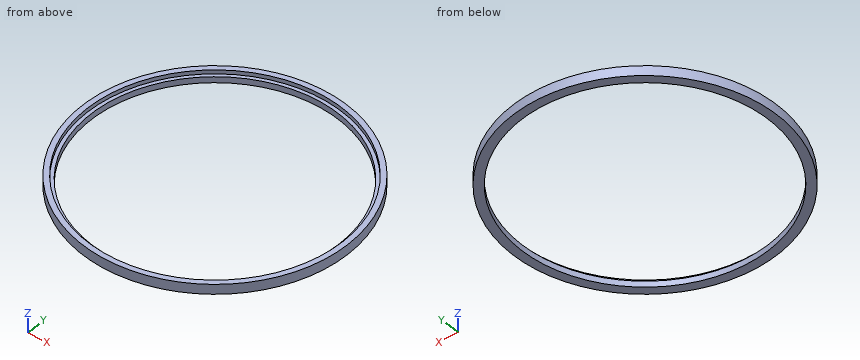
```python
from build123d import *

# Parameters (mm, degrees)
F0_R     = 67
F0_R_2   = 64.375
F1_DEPTH = 5
F0_R_3   = 62.625
F2_DEPTH = 3
F0_R_4   = 58.875
F3_DEPTH = 2
F4_R     = 5.75
F5_DEPTH = 192


# Not quite as in the source:
# - an extrude ends at something that could not be found from the text; its depth is read off the source's solid


with BuildPart() as f1:
    # F0 (on Top) → F1 (new body)
    with BuildSketch(Plane.XY):
        Circle(F0_R)
        Circle(F0_R_2, mode=Mode.SUBTRACT)
    extrude(amount=F1_DEPTH)

    # F0 (on Top) → F2 (join)
    with BuildSketch(Plane.XY):
        Circle(F0_R_2)
        Circle(F0_R_3, mode=Mode.SUBTRACT)
    extrude(amount=F2_DEPTH)

    # F0 (on Top) → F3 (cut)
    with BuildSketch(Plane.XY):
        Circle(F0_R_3)
        Circle(F0_R_4, mode=Mode.SUBTRACT)
    extrude(amount=F3_DEPTH, mode=Mode.SUBTRACT)

    # F4 (on Top) → F5 (cut, through all)
    with BuildSketch(Plane.XY):
        with Locations((0, 46.25)):
            Circle(F4_R)
    extrude(amount=-F5_DEPTH, mode=Mode.SUBTRACT)


solid = f1.part
```
Can you work these out from the model? Positions are in its coordinate system, mm. Coordinates: 2 decimals unless noted, no trailing zeros. Loops run counter-clockwise (first coordinate to the right, second up) from the corner with the lowest first, then second, coordinate; pieces in that order, holes last. Notation, with made-up numbers: (-26.5, 3) -> (14.5, 3) arc R16 ccw to (14.5, 11) -> close; hole circle Ø4 at (28.25, 39.5). An arc over 180 degrees is marked (long way). Answer as a JSON object with one key per item and string values.
1) Imagine slicing it at C-C (z = 1.55). Please give me the cut outline in (x, y) (3 decimals), then the cut area to 3 significant figures.
Results:
{"outline": "circle Ø134 at (0, 0); hole circle Ø125.25 at (0, 0)", "area": "1,780 mm^2"}
2) Imagine slicing it at A-A (x = 0). Please give me the cut outline in (y, z) (3 decimals), then the cut area to 4 significant figures.
Results:
{"outline": "(-67, 0) -> (-62.625, 0) -> (-62.625, 3) -> (-64.375, 3) -> (-64.375, 5) -> (-67, 5) -> close; (62.625, 0) -> (67, 0) -> (67, 5) -> (64.375, 5) -> (64.375, 3) -> (62.625, 3) -> close", "area": "36.75 mm^2"}
3) If I drill on line 1 (Y direction, x = 0, z = 3.5) (3 decimals); line 2 (Y direction, x = 0, z = 1.2) (3 decimals); line 3 (X direction, y = -41, z = 1.7), over which ranges is the centre line in solid material (lowest first)?
Results:
{"line 1": "y = -67 to -64.375, 64.375 to 67", "line 2": "y = -67 to -62.625, 62.625 to 67", "line 3": "x = -52.99 to -47.34, 47.34 to 52.99"}
4) For P1, Ø2, axis at x = 39, z = 1.5, coming from the -Y side; P2, Ø3, axis at x = 8.5, z = 3.5, coming from the +Y side; P3, Ø1.5, axis at y = -25.5, z = 3, coming from the +X side, each with a flat end and sliding along its axis, tell me the tip position at first contact or that it passes through.
Results:
{"P1": "stops at y = -55.18", "P2": "stops at y = 66.63", "P3": "stops at x = 62.26"}
